Work out the finished part from the listing and answer in its coordinate system (mm). A direction names the side the tool comes from. Round coordinates to 2 decimals unless told otherwise and drop trailing zeros. Order: outer loops, then holes, each group sorted by start corner. A loop starts at its lowest first (then second) coordinate and runs counter-clockwise, first axis right, second up. Notation, with made-up numbers: (69.25, 5) - (117.25, 5) arc R25 ccw to (117.25, 36) - close; hole circle Ø3 at (3.5, -38.75). An arc over 180 degrees is marked (long way). Use one line per item in the form item = value. Start each with the question number.
Q1. The part is cut by section A-A on y = 10. Determine the outline of the cut face in (x, z), plus the area to 3 significant figures.
Q2. The part is cut by section D-D on z = 7.5. State how many separate pieces and enclosed holes the cut face has, plus the area to 3 significant figures.
Q3. The part is cut by section C-C on y = 22. Determine the outline of the cut face in (x, z), plus the area to 3 significant figures.
Q4. For a pull along Y with two mould halves and no side action, classify faces 1 (the flat face through (0, 4, 0)), 2 (the cylindrical face through (-32.005, 22.946, 7.395)), 3 (the cylindrical face through (25, 63, 8)), 4 (the cylindrical face through (18.685, -5.558, 7.605)) as +Y half, -Y half, draft (parallel to the pull), parting line (faces both ways), or undercut.
Q5. Which of the six approach directions +Z, -Z, +X, -X, +Y, -Y give full straight-line access (tool end or side, diameter ignored) to faces 5 (the flat face through (-1.2, 2, 5)), 6 (the flat face through (-27, -20, 7)), 7 (the flat face through (-24, 34, 7)), 8 (the cylindrical face through (0.78, 3.48, 5.02)), 9 (the cylindrical face through (20, -18, 8))?
Q6. Given P1, Ø5, axis at x = 29, y = 57, coming from the -Z side; P2, Ø3, axis at x = -10.5, z = 5, coming from the +Y side; P3, Ø4, axis at x = 11, z = 4.5, coming from the -Y side; P4, Ø7, axis at x = 0, z = 7.5, coming from the -Y side, each flat-ended and moving along its own axis, determine where each tip first touches the part or whether it passes through.
Q7. Find the intervals of material crossed by line 1 (X direction, y = 15.5, z = 6); line 2 (X direction, y = -11, z = 0.75); line 3 (X direction, y = 20, z = 1.5), in increasing order. Write a range as [from, to].
Q8. The part is cut by section B-B on x = 0. Determine the outline of the cut face in (y, z).
from build123d import *

# Parameters (mm, degrees)
ESQUISSE1_R             = 3.15
BOSS_EXTRU_1_DEPTH      = 15
CONG_1_R                = 3
CONG_2_R                = 5
CONG_1_OF_SYM_TRIE2_R   = 3
CONG_2_OF_SYM_TRIE2_R   = 5
ESQUISSE3_R             = 5.75
ENL_V_MAT_EXTRU_1_DEPTH = 2
ENL_V_MAT_EXTRU_2_REACH = 75.144
ESQUISSE4_R             = 2.6


with BuildPart() as part:
    # Esquisse1 → Boss.-Extru.1 (new body)
    with BuildSketch(Plane.XY):
        Polygon((0, 0), (0, 5), (24, 5), (24, 65), (34, 65), (34, -20), (19, -20), (19, -5.425258757), (12, 0), align=None)
        with Locations((29, 57)):
            Circle(ESQUISSE1_R, mode=Mode.SUBTRACT)
        with Locations((26.5, -15)):
            Circle(ESQUISSE1_R, mode=Mode.SUBTRACT)
        with Locations((29, 22)):
            Circle(ESQUISSE1_R, mode=Mode.SUBTRACT)
    boss_extru_1 = extrude(amount=BOSS_EXTRU_1_DEPTH)

    # Congé1
    cong_1_edges = [part.edges().sort_by_distance(p)[0] for p in [
        (24, 5, 7.5),
        (19, -5.425258757, 7.5),
        (12, 0, 7.5),
    ]]
    fillet(cong_1_edges, radius=CONG_1_R)

    # Congé2
    cong_2_edges = [part.edges().sort_by_distance(p)[0] for p in [
        (19, -20, 7.5),
        (34, -20, 7.5),
        (24, 65, 7.5),
        (34, 65, 7.5),
    ]]
    fillet(cong_2_edges, radius=CONG_2_R - 0.0001)  # a hair under: the kernel refuses the full size

    # Symétrie2: Boss.-Extru.1 across plane
    add(boss_extru_1.mirror(Plane(origin=(0, 0, 15), x_dir=(0, 0, 1), z_dir=(1, 0, 0))))

    # Congé1 of Symétrie2
    cong_1_of_sym_trie2_edges = [part.edges().sort_by_distance(p)[0] for p in [
        (-24, 5, 7.5),
        (-19, -5.425258757, 7.5),
        (-12, 0, 7.5),
    ]]
    fillet(cong_1_of_sym_trie2_edges, radius=CONG_1_OF_SYM_TRIE2_R)

    # Congé2 of Symétrie2
    cong_2_of_sym_trie2_edges = [part.edges().sort_by_distance(p)[0] for p in [
        (-19, -20, 7.5),
        (-34, -20, 7.5),
        (-24, 65, 7.5),
        (-34, 65, 7.5),
    ]]
    fillet(cong_2_of_sym_trie2_edges, radius=CONG_2_OF_SYM_TRIE2_R - 0.0001)  # a hair under: the kernel refuses the full size

    # Esquisse3 → Enlèv. mat.-Extru.1 (cut)
    with BuildSketch(Plane.XZ):
        with Locations(Location((0, 7.5, 0), (0, 0, 270))):
            Circle(ESQUISSE3_R)
    extrude(amount=-ENL_V_MAT_EXTRU_1_DEPTH, mode=Mode.SUBTRACT)

    # Esquisse4 → Enlèv. mat.-Extru.2 (cut, up to next)
    with BuildSketch(Plane.XZ.offset(-2), mode=Mode.PRIVATE) as enl_v_mat_extru_2_sk1:
        with Locations(Location((0, 7.5, 0), (0, 0, 270))):
            Circle(ESQUISSE4_R)
    enl_v_mat_extru_2_tool1 = extrude(enl_v_mat_extru_2_sk1.sketch, amount=-ENL_V_MAT_EXTRU_2_REACH, mode=Mode.PRIVATE) & part.part
    enl_v_mat_extru_2 = enl_v_mat_extru_2_tool1.solids().sort_by_distance((0, 2, 7.5))[0]
    add(enl_v_mat_extru_2, mode=Mode.SUBTRACT)

    # Symétrie1: Enlèv. mat.-Extru.2 across Right Plane
    add(enl_v_mat_extru_2.mirror(Plane(origin=(0, 0, 0), x_dir=(0, 0, -1), z_dir=(1, 0, 0))), mode=Mode.SUBTRACT)


solid = part.part
Found:
q1.outline = (-34, 0) - (-24, 0) - (-24, 15) - (-34, 15) - close; (24, 0) - (34, 0) - (34, 15) - (24, 15) - close
q1.area = 300 mm²
q2.separate_pieces = 2
q2.enclosed_holes = 6
q2.area = 1,910 mm²
q3.outline = (-34, 0) - (-32.15, 0) - (-32.15, 15) - (-34, 15) - close; (-25.85, 0) - (-24, 0) - (-24, 15) - (-25.85, 15) - close; (24, 0) - (25.85, 0) - (25.85, 15) - (24, 15) - close; (32.15, 0) - (34, 0) - (34, 15) - (32.15, 15) - close
q3.area = 111 mm²
q4.face_1 = draft
q4.face_2 = undercut
q4.face_3 = +Y half
q4.face_4 = -Y half
q5.face_5 = -Y
q5.face_6 = +Z, -Z, +X, -X, -Y
q5.face_7 = +Z, -Z, +Y
q5.face_8 = +Y, -Y
q5.face_9 = +Z, -Z, -Y
q6.P1 = through
q6.P2 = 5
q6.P3 = -0.78
q6.P4 = 2
q7.line_1 = [-34, -24], [24, 34]
q7.line_2 = [-34, -19], [19, 34]
q7.line_3 = [-34, -31.43], [-26.57, -24], [24, 26.57], [31.43, 34]
q8.outline = (0, 0) - (5, 0) - (5, 4.9) - (2, 4.9) - (2, 1.75) - (0, 1.75) - close; (0, 13.25) - (2, 13.25) - (2, 10.1) - (5, 10.1) - (5, 15) - (0, 15) - close
